```python
from build123d import *

# Parameters (mm, degrees)
F0_R     = 35
F1_DEPTH = 180
F2_R     = 15
F3_DEPTH = 15
F4_R     = 5
F5_SIZE  = 16
F6_R     = 17.5
F7_DEPTH = 5
F8_T     = -2.5


with BuildPart() as f1:
    # F0 (on Top) → F1 (new body)
    with BuildSketch(Plane.XY):
        Circle(F0_R)
    extrude(amount=F1_DEPTH)

    # F2 (on face) → F3 (join)
    with BuildSketch(Plane.XY.offset(180)):
        Circle(F2_R)
    extrude(amount=F3_DEPTH)

    # F4
    f4_edges = [f1.edges().sort_by_distance(p)[0] for p in [
        (-35, 0, 0),
    ]]
    fillet(f4_edges, radius=F4_R)

    # F5
    f5_edges = [f1.edges().sort_by_distance(p)[0] for p in [
        (-35, 0, 180),
    ]]
    chamfer(f5_edges, length=F5_SIZE)

    # F6 (on face) → F7 (cut)
    with BuildSketch(Plane(origin=(0, 0, 0), x_dir=(1, 0, 0), z_dir=(0, 0, -1))):
        Circle(F6_R)
    extrude(amount=-F7_DEPTH, mode=Mode.SUBTRACT)

    # F8
    f8_openings = [f1.faces().sort_by_distance(p)[0] for p in [
        (0, 0, 195),
    ]]
    offset(amount=F8_T, openings=f8_openings, kind=Kind.INTERSECTION)


solid = f1.part
```
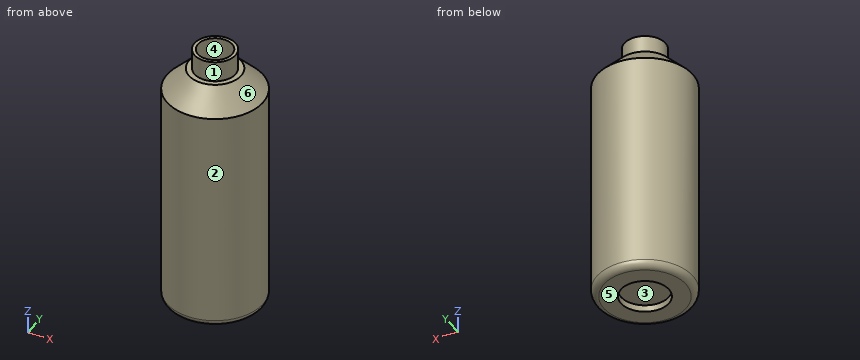
Model file for the job. Use its own axes, mm. Face numbers are marked on the shaded views. A direction names the side the tool comes from. Coordinates: 2 decimals unless noted, no trailing zeros. Write each loop counter-clockwise with the first axis right and the second up, starting at its lowest first coordinate (ties: lowest second). Pieces come first, ordered by that corner, then holes. Notation, with made-up numbers: (48, -40) - (66, -40) arc R23 cw to (66, -24) - close; hole circle Ø3 at (-36.75, 26.25). An arc over 180 degrees is marked (long way). One line per item, written item: value. Start each with the question number.
1. Slice it at C-C (z = 135.5). Write the cut outline in (x, y).
2. Probe line 1 (Z direction, x = -14, y = 6); line 2 (Y direction, x = 0, z = 183.5); line 3 (Z direction, x = -8, y = -11). List the from-to ranges inside material, lowest first. Write a range as from..to.
3. Flat gauge pins, fed straight in: pin 1 (1.5 mm diameter, centred on x = -9.5, z = 51.5, fed in from +Y); pin 2 (5 mm diameter, centred on x = 1.5, y = 2.5, fed in from -Z); pin 3 (12 mm diameter, centred on x = -20.5, z = 31, fed in from +Y). Where does each tip first touch, or does it go through?
4. Mould opens along Y. For the marked faces 4, 5 and 6 say: released by +Y, released by -Y, zero draft, split by the parting line, or undercut.
5. Tool access for the marked faces 1, 2 and 3: list every direction of +Z, -Z, +X, -X, +Y, -Y with a clear straight run to the whole face (end or side of a thin tool).
Answers below:
1. outline: circle Ø70 at (0, 0); hole circle Ø65 at (0, 0)
2. line 1: z = 5..7.5, 177.5..180
2. line 2: y = -15..-12.5, 12.5..15
2. line 3: z = 5..7.5, 177.5..195
3. pin 1: stops at y = 33.89
3. pin 2: stops at z = 5
3. pin 3: stops at y = 31.86
4. face 4: undercut
4. face 5: zero draft
4. face 6: split by the parting line
5. face 1: +Z
5. face 2: +Z, -Z
5. face 3: -Z
